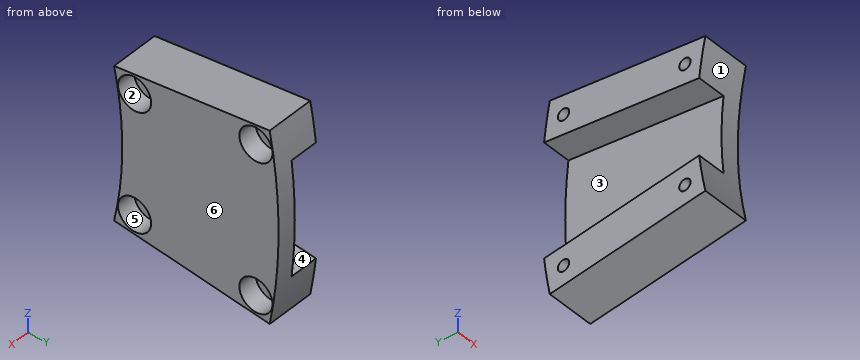
Autodesk Inventor part; units mm, degrees
ref_plane "YZ Plane" through (0, 0, 0) normal (1, 0, 0) x (0, 1, 0)
ref_plane "XZ Plane" through (0, 0, 0) normal (0, 1, 0) x (-1, 0, 0)
ref_plane "XY Plane" through (0, 0, 0) normal (0, 0, 1) x (1, 0, 0)
sketch "Sketch1" plane through (0, 0, 0) normal (1, 0, 0) x (0, 1, 0)
  circle A0 centre (0, 0) radius 54
  circle A1 centre (0, 0) radius 37.5
  line L0 (37.5, 0) -> (54, 0)
  line L1 (53.066, -10) -> (36.6367, -8)
  line L2 (53.066, 10) -> (36.6367, 8)
  arc A2 (53.066, -10) -> (53.066, 10) centre (0, 0) ccw
  arc A3 (36.6367, -8) -> (36.6367, 8) centre (0, 0) ccw
  dimension "d0" = 108
  dimension "d1" = 75
  dimension "d2" = 10
  dimension "d3" = 0
  dimension "d4" = 8
extrude "Extrusion1" add sketch "Sketch1" along normal blind 5 contours L0 A1 L2 A0 | A0 L1 A1 L0
sketch "Sketch2" plane through (0, 0, 0) normal (-1, 0, 0) x (0, 0, 1)
  arc A0 (10, 53.066) -> (-10, 53.066) centre (0, 0) ccw
  line L0 (-6, 53.6656) -> (-4, 37.2861)
  arc A1 (8, 36.6367) -> (-8, 36.6367) centre (0, 0) ccw
  line L1 (0, 54) -> (0, 37.5)
  line L2 (6, 53.6656) -> (4, 37.2861)
  arc A2 (6, 53.6656) -> (-6, 53.6656) centre (0, 0) ccw
  arc A3 (4, 37.2861) -> (-4, 37.2861) centre (0, 0) ccw
  point P0 (0, 0)
  dimension "d7" = 4
  dimension "d8" = 4
extrude "Extrusion2" cut sketch "Sketch2" against normal blind 3
sketch "Sketch3" plane through (5, 0, 0) normal (1, 0, 0) x (0, 0, -1)
  line L0 (-10, 53.066) -> (-8, 36.6367)
  circle A0 centre (0, 0) radius 52.2
  circle A1 centre (0, 0) radius 39.3
  circle A2 centre (-7.8083, 51.6127) radius 0.6
  circle A3 centre (-6.2486, 38.8001) radius 0.6
  line L1 (0, 54) -> (0, 37.3718)
  circle A4 centre (7.8083, 51.6127) radius 0.6
  circle A5 centre (6.2486, 38.8001) radius 0.6
  dimension "d15" = 104.4
  dimension "d16" = 78.6
  dimension "d17" = 1.2
  dimension "d18" = 1.2
  dimension "d19" = 2
  dimension "d20" = 2
extrude "Extrusion3" cut sketch "Sketch3" against normal through all contours A2 A0 | A0 A2 | A3 A1 | A1 A3 | A4 A0 | A0 A4 | A5 A1 | A1 A5
sketch "Sketch4" plane through (5, 0, 0) normal (1, 0, 0) x (0, 0, -1)
  circle A0 centre (-7.8083, 51.6127) radius 0.6
  circle A1 centre (-7.8083, 51.6127) radius 1.75
  circle A2 centre (7.8083, 51.6127) radius 0.6
  circle A3 centre (7.8083, 51.6127) radius 1.75
  circle A4 centre (6.2486, 38.8001) radius 0.6
  circle A5 centre (6.2486, 38.8001) radius 1.75
  circle A6 centre (-6.2486, 38.8001) radius 0.6
  circle A7 centre (-6.2486, 38.8001) radius 1.75
  point P0 (0, 0)
  dimension "d23" = 3.5
  dimension "d24" = 3.5
  dimension "d25" = 3.5
  dimension "d26" = 3.5
extrude "Extrusion4" cut sketch "Sketch4" against normal blind 2
properties part number "32111_Lock Wedge Backing_V1" material "Acetal Resin, White"
Read the model definition and answer for the solid it produces. Units are mm, in the model's axes. Face numbers are marked on the shaded views. A direction names the side the tool comes from. Coordinates: 2 decimals unless noted, no trailing zeros. Order: outer loops, then holes, each group sorted by start corner. A loop starts at its lowest first (then second) coordinate and runs counter-clockwise, first axis right, second up. Notation, with made-up numbers: M 47,3.25 L 61,3.25 A11 cw 61,23.25 Z; hole C -31,20.25 d2. An arc over 180 degrees is marked long. Put each result on its own line as item: value. Start each with the question number.
Item 1: The mould has two halves that part along Y. Classify the marked faces 1, 2 and 3: +Y half, -Y half, draft (parallel to the pull), parting line (faces both ways), or undercut.
Item 2: Given pin 1 Ø4 at (y, z) = (51, 8) entering from +X; pin 2 Ø1.5 at (x, z) = (3.5, 2) entering from -Y; pin 3 Ø1.1 at (y, z) = (51.61, 7.81) entering from -X; pin 4 Ø1.5 at (y, z) = (40, 1.5) entering from -X, each flat-ended and moving along its own axis, determine where each tip first touches the part or whether it passes through.
Item 3: Section A-A, the plane x = 2.6 is taken. Determine the outline of the cut face in (y, z).
Item 4: Consider probe 1 along Z at (x, y) = (3.6, 50.5); probe 2 along X at (y, z) = (51.25, 9); probe 3 along X at (y, z) = (52, 2). Determine where each line is inside the solid, lowest interval first. Write a range as [from, to].
Item 5: Section B-B, the plane z = 7.75 is taken. Determine the outline of the cut face in (x, y).
Item 6: For the marked faces 4, 5 and 6, determine the directions among +Z, -Z, +X, -X, +Y, -Y from which every point of the face is accessible in a straight line to the end or side of a thin tool.
Item 7: Section D-D, the plane y = 46.25 is taken. Determine the outline of the cut face in (x, z), plus the area to 3 significant figures.
Item 8: Section C-C, the plane x = 3.95 is taken. Determine the outline of the cut face in (y, z), plus the area to 3 significant figures.
Computed:
1. face 1: -Y half
1. face 2: undercut
1. face 3: draft
2. pin 1: stops at x = 5
2. pin 2: stops at y = 37.4
2. pin 3: passes through
2. pin 4: stops at x = 3
3. outline: M 36.64,-8 L 53.07,-10 A54 ccw 53.67,-6 L 37.29,-4 A37.5 cw Z; M 36.64,8 A37.5 cw 37.29,4 L 53.67,6 A54 ccw 53.07,10 Z; hole C 38.8,-6.25 d1.2; hole C 38.8,6.25 d1.2; hole C 51.61,-7.81 d1.2; hole C 51.61,7.81 d1.2
4. probe 1: z = [-9.69, -9.16], [-6.46, 6.46], [9.16, 9.69]
4. probe 2: x = [0, 3]
4. probe 3: x = [3, 5]
5. outline: M 0,36.69 L 5,36.69 L 5,37.9 L 3,37.9 L 3,39.7 L 5,39.7 L 5,49.86 L 3,49.86 L 3,51.02 L 0,51.02 Z; M 0,52.21 L 3,52.21 L 3,53.36 L 5,53.36 L 5,53.44 L 0,53.44 Z
6. face 4: -X, +Y
6. face 5: +X
6. face 6: +Z, -Z, +X, +Y, -Y
7. outline: M 0,-9.17 L 5,-9.17 L 5,9.17 L 0,9.17 L 0,5.09 L 3,5.09 L 3,-5.09 L 0,-5.09 Z
7. area: 61.1 mm2
8. outline: M 36.64,-8 L 53.07,-10 A54 ccw 53.07,10 L 36.64,8 A37.5 cw Z; hole C 38.8,-6.25 d3.5; hole C 38.8,6.25 d3.5; hole C 51.61,-7.81 d3.5; hole C 51.61,7.81 d3.5
8. area: 260 mm2
